Part model, mm, in its own coordinate system. A direction names the side the tool comes from. Coordinates: 2 decimals unless noted, no trailing zeros. Use a Markdown table: item, result. Add a question column.
1. Wall check: probe 1 along Z at (x, y) = (0.75, 56); probe 2 along Z at (x, y) = (-0.45, -40.5); probe 3 along Z at (x, y) = (-1.8, 29.5). Give the ranges that are in metal, low to high. Write a range as [from, to].
2. Band-saw the part on A-A, the plane x = 0.35. Count the separate pieces of the cut face and the enclosed holes in it, plus the area to 3 significant figures.
3. Pull direction Y, two halves, no side cores. Call faces 3 (the flat face through (2, -21, 46)), 4 (the cylindrical face through (0.028, 72.163, 53.302)): pulls with the +Y half, pulls with the -Y half, needs draft (parallel to the pull), parting line crosses it, or undercut.
4. Drop flat-ended pins along their axis: pin 1 (5 mm diameter, centred on y = -76.81, z = 16.72, fed in from -X) (3 decimals); pin 2 (1 mm diameter, centred on x = -0.5, y = -26, fed in from -Z); pin 3 (16 mm diameter, centred on y = 0, z = -35, fed in from -X); pin 4 (12 mm diameter, centred on y = 46, z = -9.5, fed in from -X). Give the stop position or say it passes through.
5. 3-axis set-ups, long thin cutter, end or side, ignore diameter. For faces 1 (the flat face through (-1, -10.4, 22.9)), 2 (the cylindrical face through (0, 18, -24)): which of +Z, -Z, +X, -X, +Y, -Y reach the whole face in a straight line?
from build123d import *

# Parameters (mm, degrees)
SKETCH1_R           = 100
SKETCH1_R_2         = 50
BOSS_EXTRUDE1_DEPTH = 2
SKETCH1_3_R         = 50
SKETCH1_3_R_2       = 25
BOSS_EXTRUDE2_DEPTH = 1
SKETCH1_4_R         = 5
CUT_EXTRUDE1_DEPTH  = 142.435497666
CIRPATTERN1_COUNT   = 5
SKETCH2_R           = 3
CUT_EXTRUDE2_DEPTH  = 142.477913471
CIRPATTERN2_COUNT   = 10


with BuildPart() as part:
    # Sketch1 → Boss-Extrude1 (new, symmetric)
    with BuildSketch(Plane.YZ):
        with Locations(Location((0, 0, 0), (0, 0, 270))):
            Circle(SKETCH1_R)
        with Locations(Location((0, 0, 0), (0, 0, 270))):
            Circle(SKETCH1_R_2, mode=Mode.SUBTRACT)
    extrude(amount=BOSS_EXTRUDE1_DEPTH, both=True)

    # Sketch1_3 → Boss-Extrude2 (add, symmetric)
    with BuildSketch(Plane.YZ):
        with Locations(Location((0, 0, 0), (0, 0, 270))):
            Circle(SKETCH1_3_R)
        with Locations(Location((0, 0, 0), (0, 0, 270))):
            Circle(SKETCH1_3_R_2, mode=Mode.SUBTRACT)
    extrude(amount=BOSS_EXTRUDE2_DEPTH, both=True)

    # Sketch1_4 → Cut-Extrude1 (cut, symmetric)
    with BuildSketch(Plane.YZ):
        with BuildLine():
            ThreePointArc((6.128110462, 29.367435403), (12.044034772, 33.240656227), (8.170813949, 39.156580538))
            ThreePointArc((8.170813949, 39.156580538), (0, 40), (-8.170813949, 39.156580538))
            ThreePointArc((-8.170813949, 39.156580538), (-12.044034772, 33.240656227), (-6.128110462, 29.367435403))
            ThreePointArc((-6.128110462, 29.367435403), (0, 30), (6.128110462, 29.367435403))
        make_face()
        with Locations(Location((0, -35, 0), (0, 0, 270))):
            Circle(SKETCH1_4_R)
    cut_extrude1 = extrude(amount=CUT_EXTRUDE1_DEPTH, both=True, mode=Mode.SUBTRACT)

    # CirPattern1: Cut-Extrude1 ×5 about axis
    cirpattern1_axis = Axis((0, 0, 0), (1, 0, 0))
    for i in range(1, CIRPATTERN1_COUNT):
        add(cut_extrude1.rotate(cirpattern1_axis, i * 360 / CIRPATTERN1_COUNT), mode=Mode.SUBTRACT)

    # Sketch2 → Cut-Extrude2 (cut, symmetric)
    with BuildSketch(Plane.YZ.offset(2)):
        with BuildLine():
            ThreePointArc((3, 58), (0.00012401, 60.999999997), (-2.99999999, 58.000248019))
            ThreePointArc((-2.99999999, 58.000248019), (-0.000124015, 55.000551153), (2.999999944, 58))
        make_face()
        with Locations(Location((-27.245072384, 87.873238422, 0), (0, 0, 270))):
            Circle(SKETCH2_R)
        with Locations(Location((-16.636821514, 84.859364489, 0), (0, 0, 270))):
            Circle(SKETCH2_R)
        with Locations(Location((-7.834358076, 78.215942177, 0), (0, 0, 270))):
            Circle(SKETCH2_R)
        with Locations(Location((-2.027172867, 68.840707643, 0), (0, 0, 270))):
            Circle(SKETCH2_R)
    cut_extrude2 = extrude(amount=CUT_EXTRUDE2_DEPTH, both=True, mode=Mode.SUBTRACT)

    # CirPattern2: Cut-Extrude2 ×10 about axis
    cirpattern2_axis = Axis((0, 0, 0), (1, 0, 0))
    for i in range(1, CIRPATTERN2_COUNT):
        add(cut_extrude2.rotate(cirpattern2_axis, i * 360 / CIRPATTERN2_COUNT), mode=Mode.SUBTRACT)


solid = part.part
Geometry check:
| question | item | result |
|---|---|---|
| 1 | probe 1 | z = [-82.85, -20.8], [-15.04, 15.04], [20.8, 82.85] |
| 1 | probe 2 | z = [-91.43, -70.76], [-65.01, -59.37], [-54.4, 51.97], [57.04, 91.43] |
| 1 | probe 3 | z = [-95.55, -89.85], [-85.89, -40.37], [40.37, 84.11], [90.1, 95.55] |
| 2 | separate pieces | 1 |
| 2 | enclosed holes | 61 |
| 2 | area | 26,500 mm^2 |
| 3 | face 3 | needs draft |
| 3 | face 4 | undercut |
| 4 | pin 1 | passes through |
| 4 | pin 2 | stops at z = -96.69 |
| 4 | pin 3 | stops at x = -1 |
| 4 | pin 4 | stops at x = -2 |
| 5 | face 1 | -X |
| 5 | face 2 | +X, -X |
